Design review of the part built by this model. Coordinates are the model's own, in mm. Face numbers are marked on the shaded views. Coordinates: 2 decimals unless noted, no trailing zeros. Loops run counter-clockwise (first coordinate to the right, second up) from the corner with the lowest first, then second, coordinate; pieces in that order, holes last.
Q1. Add section D-D on x = -3.5. Give the boundary of the cut face in (y, z).
Q2. Add section A-A on y = 0. Give the boundary of the cut face in (x, z), and give its area (3 significant figures).
Q3. For P1, Ø3.5, axis at x = 0, y = 0, coming from the -Z side; P2, Ø1.5, axis at y = 3.5, z = 6, coming from the +X side; P3, Ø1, axis at y = 1, z = 13, coming from the -X side; P4, Ø1.5, axis at x = -4, z = 5, coming from the +Y side, all flat-tipped, find the tip position at first contact; note any pin that passes through.
Q4. Draft analysis for pull direction Y (two halves, no side actions). For the marked faces 1, 2 and 3, state which applies: released by +Y, released by -Y, zero draft, split by the parting line, or undercut.
Q5. Wall thickness on probe 1 along Z at (x, y) = (-2.5, 5.25); probe 2 along Y at (x, z) = (0, 6.5); probe 3 along Y at (x, z) = (1.25, 7.5): over which ranges is each line inside the solid? List them lowest first.
Q6. Add section C-C on z = 10.25. Give the boundary of the cut face in (x, y), and give its area (3 significant figures).
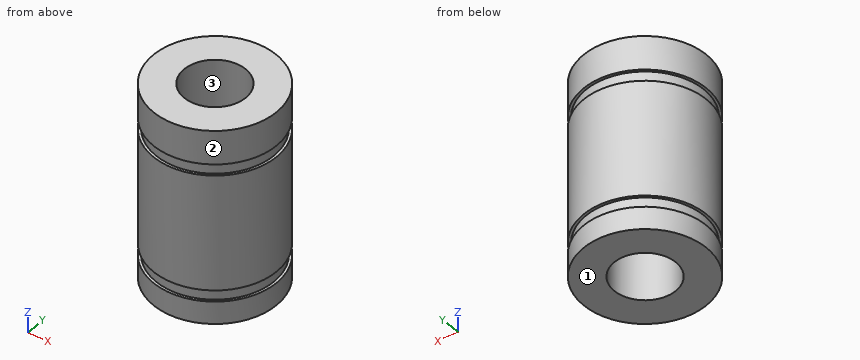
```python
from build123d import *

# Parameters (mm, degrees)
SKETCH1_R           = 6
SKETCH1_R_2         = 3
BOSS_EXTRUDE1_DEPTH = 19
SKETCH2_W           = 1.849781756
SKETCH2_H           = 1.1


with BuildPart() as part:
    # Sketch1 → Boss-Extrude1 (new body)
    with BuildSketch(Plane.XY):
        Circle(SKETCH1_R)
        Circle(SKETCH1_R_2, mode=Mode.SUBTRACT)
    extrude(amount=BOSS_EXTRUDE1_DEPTH)

    # Sketch2 → Cut-Revolve1 (revolve, cut)
    with BuildSketch(Plane(origin=(0, 0, 0), x_dir=(1, 0, 0), z_dir=(0, 1, 0))):
        with Locations((6.674890878, -2.75)):
            Rectangle(SKETCH2_W, SKETCH2_H)
        with Locations((6.674890878, -15.15)):
            Rectangle(SKETCH2_W, SKETCH2_H)
    revolve(axis=Axis((0, 0, 0), (0, 0, 1)), mode=Mode.SUBTRACT)


solid = part.part
```
Entries:
1. outline: (-4.87, 0) - (4.87, 0) - (4.87, 2.2) - (4.56, 2.2) - (4.56, 3.3) - (4.87, 3.3) - (4.87, 14.6) - (4.56, 14.6) - (4.56, 15.7) - (4.87, 15.7) - (4.87, 19) - (-4.87, 19) - (-4.87, 15.7) - (-4.56, 15.7) - (-4.56, 14.6) - (-4.87, 14.6) - (-4.87, 3.3) - (-4.56, 3.3) - (-4.56, 2.2) - (-4.87, 2.2) - close
2. outline: (-6, 0) - (-3, 0) - (-3, 19) - (-6, 19) - (-6, 15.7) - (-5.75, 15.7) - (-5.75, 14.6) - (-6, 14.6) - (-6, 3.3) - (-5.75, 3.3) - (-5.75, 2.2) - (-6, 2.2) - close; (3, 0) - (6, 0) - (6, 2.2) - (5.75, 2.2) - (5.75, 3.3) - (6, 3.3) - (6, 14.6) - (5.75, 14.6) - (5.75, 15.7) - (6, 15.7) - (6, 19) - (3, 19) - close
2. area: 113 mm2
3. P1: passes through
3. P2: stops at x = 5.33
3. P3: stops at x = -5.98
3. P4: stops at y = 5.04
4. face 1: zero draft
4. face 2: split by the parting line
4. face 3: undercut
5. probe 1: z = 0 to 2.2, 3.3 to 14.6, 15.7 to 19
5. probe 2: y = -6 to -3, 3 to 6
5. probe 3: y = -5.87 to -2.73, 2.73 to 5.87
6. outline: circle Ø12 at (0, 0); hole circle Ø6 at (0, 0)
6. area: 84.8 mm2
